Can you work these out from the drawing? Everything is in mm from the part's minimum corner. A direction names the side the tool comes from. Coordinates: 2 decimals unless noted, no trailing zeros. Order: outer loops, then holes, each group sorted by start corner. A loop starts at its lowest first (then second) coordinate and runs counter-clockwise, first axis right, second up. Notation, with made-up numbers: (50.25, 71) -> (54.25, 71) arc R31 cw to (54.25, 105) -> close; hole circle Ø2 at (16, 18). An arc over 180 degrees is marked (long way). Answer in a Markdown table with one row per item.
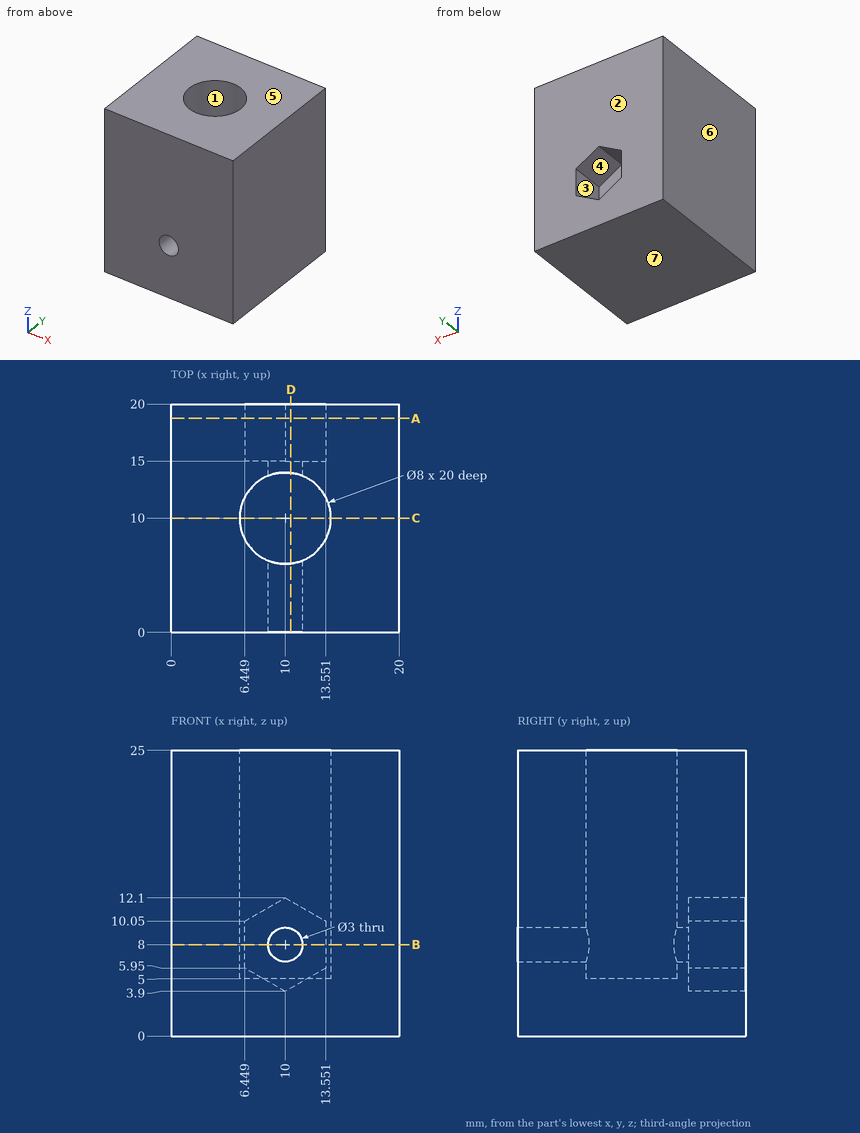
(1) Suppose I cut it at B-B (z = 8). Please give me the cut outline in (x, y).
Response values:
| item | result |
|---|---|
| outline | (0, 0) -> (8.5, 0) -> (8.5, 6.29) arc R4 cw to (8.5, 13.71) -> (8.5, 15) -> (6.45, 15) -> (6.45, 20) -> (0, 20) -> close; (11.5, 0) -> (20, 0) -> (20, 20) -> (13.55, 20) -> (13.55, 15) -> (11.5, 15) -> (11.5, 13.71) arc R4 cw to (11.5, 6.29) -> close |
(2) On a 3-axis mill with a long thin cutter (end or side, diameter ignored), from which of +Z, -Z, +X, -X, +Y, -Y can I reach the whole of each face in a straight line? I mean the marked faces 1, 2 and 3. Say none if no direction works.
Response values:
| item | result |
|---|---|
| face 1 | +Z |
| face 2 | +Z, -Z, +X, -X, +Y |
| face 3 | +Y |
(3) Suppose I cut it at A-A (y = 18.75). Please give me the cut outline in (x, z), and give its area (3 significant figures).
Response values:
| item | result |
|---|---|
| outline | (0, 0) -> (20, 0) -> (20, 25) -> (0, 25) -> close; hole (6.45, 5.95) -> (10, 3.9) -> (13.55, 5.95) -> (13.55, 10.05) -> (10, 12.1) -> (6.45, 10.05) -> close |
| area | 456 mm2 |
(4) Suppose I cut it at C-C (y = 10). Please give me the cut outline in (x, z).
Response values:
| item | result |
|---|---|
| outline | (0, 0) -> (20, 0) -> (20, 25) -> (14, 25) -> (14, 5) -> (6, 5) -> (6, 25) -> (0, 25) -> close |
(5) We'd pull the mould along Z, two halves only. Please class the marked faces 4, 5, 6 and 7: +Z half, -Z half, draft (parallel to the pull), parting line (faces both ways), or undercut.
Response values:
| item | result |
|---|---|
| face 4 | undercut |
| face 5 | +Z half |
| face 6 | draft |
| face 7 | -Z half |
(6) Suppose I cut it at D-D (x = 10.5). Please give me the cut outline in (y, z).
Response values:
| item | result |
|---|---|
| outline | (0, 0) -> (20, 0) -> (20, 4.19) -> (15, 4.19) -> (15, 6.59) -> (13.97, 6.59) -> (13.97, 5) -> (6.03, 5) -> (6.03, 6.59) -> (0, 6.59) -> close; (0, 9.41) -> (6.03, 9.41) -> (6.03, 25) -> (0, 25) -> close; (13.97, 9.41) -> (15, 9.41) -> (15, 11.81) -> (20, 11.81) -> (20, 25) -> (13.97, 25) -> close |
(7) Will this pin go through, and if not, where does the flat tip stop? pin 1 Ø5 at (x, z) = (10, 8) entering from +Y.
Response values:
| item | result |
|---|---|
| pin 1 | y = 15 |
(8) I need wall thicknesses on line 1 (X direction, y = 14.2, z = 8); line 2 (Z direction, x = 10, y = 14.2); line 3 (Y direction, x = 8.5, z = 21). Which ranges of each line are inside material? Lowest first, please. Write a range as [from, to].
Response values:
| item | result |
|---|---|
| line 1 | [0, 8.5], [11.5, 20] |
| line 2 | [0, 6.5], [9.5, 25] |
| line 3 | [0, 6.29], [13.71, 20] |
